Geometry check sheet. Reference: drawing and pictorial views, mm from the part's lowest x, y, z. Give positions to 0.01 mm unless a question says otherwise; leave off trailing zeros. Loops run counter-clockwise (first coordinate to the right, second up) from the corner with the lowest first, then second, coordinate; pieces in that order, holes last. Notation, with made-up numbers: (31, -2.5) -> (50, -2.5) arc R27 ccw to (50, 16.5) -> close; hole circle Ø8 at (37.25, 41). An arc over 180 degrees is marked (long way). One line per item, written item: value. Start each with the question number.
(1) Scan lines: line 1 along X through (y, z) = (4.25, 0.75); line 2 along Y through (x, z) = (4, 1.25); line 3 along X through (y, z) = (2.5, 0.7). Record each from-to range of solid material in increasing order. Write a range as from..to.
(2) Sectioned sample at D-D, the plane y = 13.25. Record the cut outline in (x, z).
(3) Draft check along X on the marked faces 1, 2 and 3. Enter one of: pulls with the +X half, pulls with the -X half, needs draft (parallel to the pull), parting line crosses it, or undercut.
(4) Sectioned sample at B-B, the plane y = 2.5. Record the cut outline in (x, z).
(5) Sectioned sample at C-C, the plane z = 0.7. Record the cut outline in (x, y), then the cut area to 3 significant figures.
(6) Sectioned sample at A-A, the plane x = 14. Record the cut outline in (y, z), then the cut area to 3 significant figures.
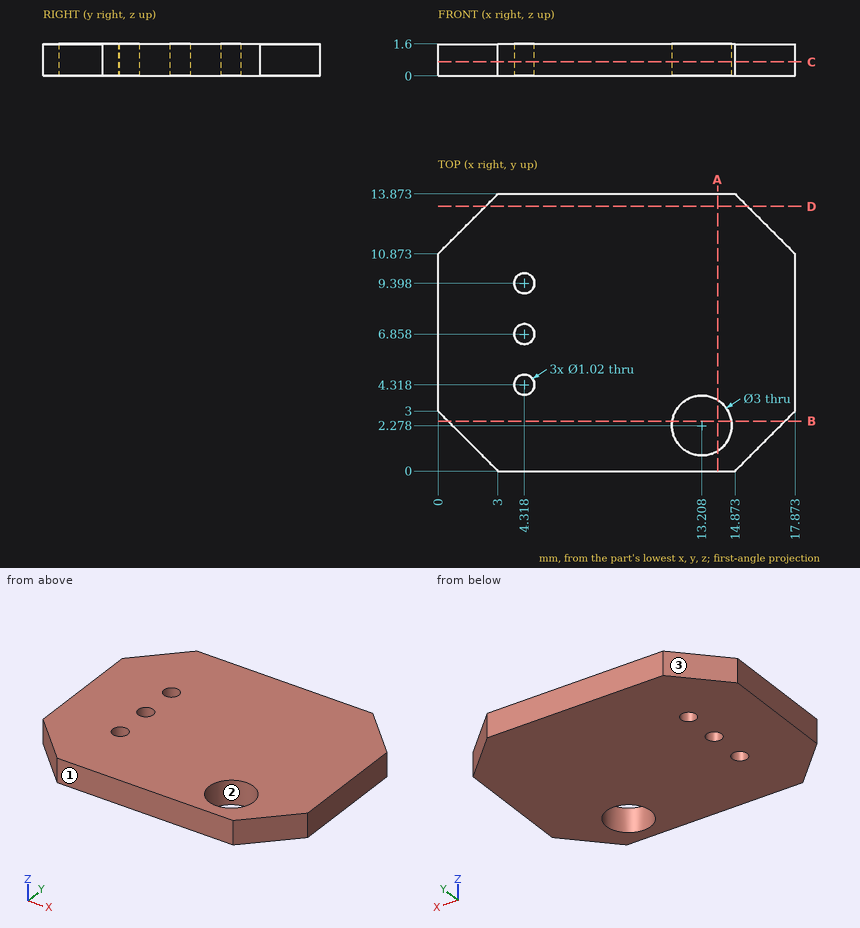
Calculated:
1. line 1: x = 0..3.81, 4.82..17.87
1. line 2: y = 0..3.92, 4.72..6.46, 7.26..9, 9.8..13.87
1. line 3: x = 0.5..11.72, 14.69..17.37
2. outline: (2.38, 0) -> (15.5, 0) -> (15.5, 1.6) -> (2.38, 1.6) -> close
3. face 1: needs draft
3. face 2: undercut
3. face 3: pulls with the -X half
4. outline: (0.5, 0) -> (11.72, 0) -> (11.72, 1.6) -> (0.5, 1.6) -> close; (14.69, 0) -> (17.37, 0) -> (17.37, 1.6) -> (14.69, 1.6) -> close
5. outline: (0, 3) -> (3, 0) -> (14.87, 0) -> (17.87, 3) -> (17.87, 10.87) -> (14.87, 13.87) -> (3, 13.87) -> (0, 10.87) -> close; hole circle Ø1.02 at (4.32, 4.32); hole circle Ø1.02 at (4.32, 6.86); hole circle Ø1.02 at (4.32, 9.4); hole circle Ø3 at (13.21, 2.28)
5. area: 220 mm2
6. outline: (0, 0) -> (1, 0) -> (1, 1.6) -> (0, 1.6) -> close; (3.55, 0) -> (13.87, 0) -> (13.87, 1.6) -> (3.55, 1.6) -> close
6. area: 18.1 mm2
